Geometry: final body of the model. Coordinates: model frame, mm. A direction names the side the tool comes from. Coordinates: 2 decimals unless noted, no trailing zeros. Loops run counter-clockwise (first coordinate to the right, second up) from the corner with the lowest first, then second, coordinate; pieces in that order, holes last. Notation, with made-up numbers: (1.25, 82.5) - (27.25, 82.5) arc R22 cw to (27.25, 102.5) - close; hole circle Ø5 at (89, 47). An arc over 180 degrees is marked (long way). Write each question's results on one line, items separated by ' | '. Start each with the question number.
from build123d import *

# Parameters (mm, degrees)
SKETCH1_R           = 1
SKETCH1_R_2         = 2.25
SKETCH1_R_3         = 1.6
BOSS_EXTRUDE1_DEPTH = 3


with BuildPart() as part:
    # Sketch1 → Boss-Extrude1 (new body)
    with BuildSketch(Plane(origin=(0, 0, 0), x_dir=(1, 0, 0), z_dir=(0, 1, 0))):
        Polygon((43.076410298, 50.123925917), (42.618597625, 48.402115535), (19.4637773, 25.158118275), (-19.4637773, 25.158118275), (-42.618597625, 48.402115535), (-45.64603124, 59.788140743), (-55.300297258, 62.394891143), (-62.384942335, 55.337426715), (-59.815321393, 45.673211889), (-50.185022628, 43.072932893), (-35, 26.288270568), (-34.873, 0), (-35, -26.288270568), (-50.185022628, -43.072932893), (-59.815321393, -45.673211889), (-62.384942335, -55.337426715), (-55.300297258, -62.394891143), (-45.64603124, -59.788140743), (-42.618597625, -48.402115535), (-19.4637773, -25.158118275), (19.4637773, -25.158118275), (42.618597625, -48.402115535), (45.64603124, -59.788140743), (55.300297258, -62.394891143), (62.384942335, -55.337426715), (59.815321393, -45.673211889), (50.185022628, -43.072932893), (35, -26.288270568), (34.873, 0), (35, 26.288270568), (50.185022628, 43.072932893), (59.815321393, 45.673211889), (62.384942335, 55.337426715), (55.300297258, 62.394891143), (45.64603124, 59.788140743), align=None)
        with Locations((-52.730676316, -57.230676316)):
            Circle(SKETCH1_R, mode=Mode.SUBTRACT)
        with Locations((-57.230676316, -52.730676316)):
            Circle(SKETCH1_R, mode=Mode.SUBTRACT)
        with Locations((-48.230676316, -52.730676316)):
            Circle(SKETCH1_R, mode=Mode.SUBTRACT)
        with Locations((-52.730676316, -48.230676316)):
            Circle(SKETCH1_R, mode=Mode.SUBTRACT)
        with Locations((-30, -17)):
            Circle(SKETCH1_R_2, mode=Mode.SUBTRACT)
        with Locations((-15.25, -15.25)):
            Circle(SKETCH1_R_3, mode=Mode.SUBTRACT)
        with Locations((52.730676316, -57.230676316)):
            Circle(SKETCH1_R, mode=Mode.SUBTRACT)
        with Locations((48.230676316, -52.730676316)):
            Circle(SKETCH1_R, mode=Mode.SUBTRACT)
        with Locations((52.730676316, -48.230676316)):
            Circle(SKETCH1_R, mode=Mode.SUBTRACT)
        with Locations((57.230676316, -52.730676316)):
            Circle(SKETCH1_R, mode=Mode.SUBTRACT)
        with Locations((30, -17)):
            Circle(SKETCH1_R_2, mode=Mode.SUBTRACT)
        with Locations((15.25, -15.25)):
            Circle(SKETCH1_R_3, mode=Mode.SUBTRACT)
        with Locations((-15.25, 15.25)):
            Circle(SKETCH1_R_3, mode=Mode.SUBTRACT)
        with Locations((-30, 17)):
            Circle(SKETCH1_R_2, mode=Mode.SUBTRACT)
        with Locations((-57.230676316, 52.730676316)):
            Circle(SKETCH1_R, mode=Mode.SUBTRACT)
        with Locations((-52.730676316, 48.230676316)):
            Circle(SKETCH1_R, mode=Mode.SUBTRACT)
        with Locations((-48.230676316, 52.730676316)):
            Circle(SKETCH1_R, mode=Mode.SUBTRACT)
        with Locations((-52.730676316, 57.230676316)):
            Circle(SKETCH1_R, mode=Mode.SUBTRACT)
        with Locations((15.25, 15.25)):
            Circle(SKETCH1_R_3, mode=Mode.SUBTRACT)
        with Locations((30, 17)):
            Circle(SKETCH1_R_2, mode=Mode.SUBTRACT)
        with Locations((52.730676316, 48.230676316)):
            Circle(SKETCH1_R, mode=Mode.SUBTRACT)
        with Locations((48.230676316, 52.730676316)):
            Circle(SKETCH1_R, mode=Mode.SUBTRACT)
        with Locations((57.230676316, 52.730676316)):
            Circle(SKETCH1_R, mode=Mode.SUBTRACT)
        with Locations((52.730676316, 57.230676316)):
            Circle(SKETCH1_R, mode=Mode.SUBTRACT)
    extrude(amount=BOSS_EXTRUDE1_DEPTH)


solid = part.part
1) Section query B-B on z = 31.5. Output: boundary loops of the cut face in (x, y).
2) Section query C-C on x = 39. Output: boundary loops of the cut face in (y, z).
3) Section query D-D on y = 1.4. Count the separate pieces of the cut face and the enclosed holes in it, and give its area (3 significant figures).
4) Section query A-A on x = -15.25. Output: boundary loops of the cut face in (y, z), and give its area (3 significant figures).
5) Material intervals for line 1 (Z direction, x = 53.5, y = 1.6); line 2 (X direction, y = 0.95, z = -15.25); line 3 (X direction, y = 1.4, z = -17), sorted ascending. Write a range as [from, to].
6) Pin query (flat end, axial travel): pin 1 Ø2.5 at (x, z) = (-52.73, 48.23) entering from -Y; pin 2 Ø1 at (y, z) = (1, 0.5) entering from +X. Return the tip coordinate at first contact, or that it passes through.
7) Access query for faces 5 (the flat face through (0, 1, -25.158)), 6 (the flat face through (61.118, 1.479, 50.573)), 7 (the flat face through (50.406, 1.479, 61.073)). Directions: +Z, -Z, +X, -X, +Y, -Y. A direction counts if a zero-diameter tool reaches every point of the face in a straight line with its end or side. Return the directions, or none.
8) Pull-direction query (Z, two-part tool) for faces 1 (the cylindrical face through (13.65, 1.48, 15.18)), 2 (the flat face through (30.88, 1.48, 36.62)), 3 (the flat face through (-44.111, 1.479, -54.015)), 4 (the flat face through (0, 0, 4)); classes: released by +Z, released by -Z, zero draft, split by the parting line, or undercut.
Returned:
1) outline: (-39.72, 0) - (-25.78, 0) - (-25.78, 3) - (-39.72, 3) - close; (25.78, 0) - (39.72, 0) - (39.72, 3) - (25.78, 3) - close
2) outline: (0, -44.77) - (3, -44.77) - (3, -30.71) - (0, -30.71) - close; (0, 30.71) - (3, 30.71) - (3, 44.77) - (0, 44.77) - close
3) separate pieces: 1 | enclosed holes: 24 | area: 5,560 mm²
4) outline: (0, -25.16) - (3, -25.16) - (3, -16.85) - (0, -16.85) - close; (0, -13.65) - (3, -13.65) - (3, 13.65) - (0, 13.65) - close; (0, 16.85) - (3, 16.85) - (3, 25.16) - (0, 25.16) - close | area: 132 mm²
5) line 1: z = [-61.91, -57.87], [-56.59, -48.87], [-47.59, -43.97], [43.97, 47.59], [48.87, 56.59], [57.87, 61.91] | line 2: x = [-34.95, -31.41], [-28.59, -16.85], [-13.65, 13.65], [16.85, 28.59], [31.41, 34.95] | line 3: x = [-34.96, -32.25], [-27.75, 27.75], [32.25, 34.96]
6) pin 1: stops at y = 0 | pin 2: stops at x = 34.88
7) face 5: -Z, +Y, -Y | face 6: +X, +Y, -Y | face 7: +Z, +Y, -Y
8) face 1: undercut | face 2: released by +Z | face 3: released by -Z | face 4: zero draft
